Could you check a few things on this model? Use its own coordinates, in mm. A direction names the side the tool comes from. Coordinates: 2 decimals unless noted, no trailing zeros. Loops run counter-clockwise (first coordinate to the right, second up) from the corner with the lowest first, then second, coordinate; pieces in that order, holes last.
1) Imagine slicing it at D-D on x = -12. Please give me the cut outline in (y, z), plus the area to 3 significant figures.
2) For faces 1 (the face through (-19.962, 22.004, -21.009)), 2 (the face through (14.53, 63.57, -16.02)), 3 (the face through (39, 7, 17)), which set-ups out of +Z, -Z, +X, -X, +Y, -Y let a thin tool reach every point of the face, with its end or its side?
3) Will these pins go through, and if not, where does the flat tip stop? P1, Ø9.5, axis at x = -21, y = 24, coming from the +Z side; P2, Ø6.5, axis at x = 15, y = 60, coming from the +Z side; P3, Ø3.5, axis at x = 15, y = 60, coming from the +Z side.
4) Thinking about a two-plate mould opening in X: for faces 4 (the face through (39, 56, 17)), 5 (the face through (41, 39, 0)), 6 (the face through (-1, 49, 5)), which applies, released by +X, released by -X, zero draft, split by the parting line, or undercut?
5) Imagine slicing it at C-C on z = 4. Please give me the cut outline in (x, y), plus the area to 3 significant figures.
6) Imagine slicing it at B-B on x = 15. Please give me the cut outline in (y, z).
7) If I drill on line 1 along Y through (x, z) = (15, -20.8); line 2 along Y through (x, z) = (-31, 4); line 3 along X through (y, z) = (32.5, 10), over which ranges is the centre line in solid material (lowest first)?
8) Imagine slicing it at A-A on y = 60. Please give me the cut outline in (x, z), plus the area to 3 significant figures.
```python
from build123d import *

# Parameters (mm, degrees)
SKETCH_1_W          = 82
SKETCH_1_H          = 48
EXTRUDE_1_DEPTH     = 80
SKETCH_2_W          = 72
SKETCH_2_H          = 44
SKETCH_2_H_2        = 22
CUT_EXTRUDE_1_DEPTH = 38
CUT_EXTRUDE_2_REACH = 84
SKETCH_3_W          = 7
SKETCH_3_H          = 4
SKETCH_5_R          = 3.6
CUT_EXTRUDE_3_DEPTH = 4.1
CUT_EXTRUDE_4_REACH = 12
SKETCH_6_R          = 2.25


with BuildPart() as part:
    # 草圖1 → 填料-伸長1 (new body)
    with BuildSketch(Plane(origin=(0, 0, 0), x_dir=(1, 0, 0), z_dir=(0, 1, 0))):
        Rectangle(SKETCH_1_W, SKETCH_1_H)
    extrude(amount=EXTRUDE_1_DEPTH)

    # 草圖2 → 除料-伸長1 (cut)
    with BuildSketch(Plane.XY.offset(24)):
        with Locations((0, 27)):
            Rectangle(SKETCH_2_W, SKETCH_2_H)
        with Locations((0, 65)):
            Rectangle(SKETCH_2_W, SKETCH_2_H_2)
    extrude(amount=-CUT_EXTRUDE_1_DEPTH, mode=Mode.SUBTRACT)

    # 草圖3 → 除料-伸長2 (cut, up to next)
    with BuildSketch(Plane(origin=(41, 0, 0), x_dir=(0, 0, -1), z_dir=(1, 0, 0)), mode=Mode.PRIVATE) as cut_extrude_2_sk1:
        with Locations((-20.5, 7)):
            Rectangle(SKETCH_3_W, SKETCH_3_H)
    cut_extrude_2_tool1 = extrude(cut_extrude_2_sk1.sketch, amount=-CUT_EXTRUDE_2_REACH, mode=Mode.PRIVATE) & part.part
    add(cut_extrude_2_tool1.solids().sort_by_distance((41, 7, 20.5))[0], mode=Mode.SUBTRACT)
    # 草圖3 → 除料-伸長2 (cut, up to next)
    with BuildSketch(Plane(origin=(41, 0, 0), x_dir=(0, 0, -1), z_dir=(1, 0, 0)), mode=Mode.PRIVATE) as cut_extrude_2_sk2:
        with Locations((-20.5, 56)):
            Rectangle(SKETCH_3_W, SKETCH_3_H)
    cut_extrude_2_tool2 = extrude(cut_extrude_2_sk2.sketch, amount=-CUT_EXTRUDE_2_REACH, mode=Mode.PRIVATE) & part.part
    add(cut_extrude_2_tool2.solids().sort_by_distance((41, 56, 20.5))[0], mode=Mode.SUBTRACT)

    # 草圖5 → 除料-伸長3 (cut)
    with BuildSketch(Plane.XY.offset(-14)):
        with Locations((-21, 60)):
            Circle(SKETCH_5_R)
        with Locations((15, 60)):
            Circle(SKETCH_5_R)
        with Locations((15, 24)):
            Circle(SKETCH_5_R)
        with Locations((-21, 24)):
            Circle(SKETCH_5_R)
    extrude(amount=-CUT_EXTRUDE_3_DEPTH, mode=Mode.SUBTRACT)

    # 草圖6 → 除料-伸長4 (cut, up to next)
    with BuildSketch(Plane.XY.offset(-14), mode=Mode.PRIVATE) as cut_extrude_4_sk1:
        with Locations((-21, 60)):
            Circle(SKETCH_6_R)
    cut_extrude_4_tool1 = extrude(cut_extrude_4_sk1.sketch, amount=-CUT_EXTRUDE_4_REACH, mode=Mode.PRIVATE) & part.part
    add(cut_extrude_4_tool1.solids().sort_by_distance((-21, 60, -14))[0], mode=Mode.SUBTRACT)
    # 草圖6 → 除料-伸長4 (cut, up to next)
    with BuildSketch(Plane.XY.offset(-14), mode=Mode.PRIVATE) as cut_extrude_4_sk2:
        with Locations((15, 60)):
            Circle(SKETCH_6_R)
    cut_extrude_4_tool2 = extrude(cut_extrude_4_sk2.sketch, amount=-CUT_EXTRUDE_4_REACH, mode=Mode.PRIVATE) & part.part
    add(cut_extrude_4_tool2.solids().sort_by_distance((15, 60, -14))[0], mode=Mode.SUBTRACT)
    # 草圖6 → 除料-伸長4 (cut, up to next)
    with BuildSketch(Plane.XY.offset(-14), mode=Mode.PRIVATE) as cut_extrude_4_sk3:
        with Locations((15, 24)):
            Circle(SKETCH_6_R)
    cut_extrude_4_tool3 = extrude(cut_extrude_4_sk3.sketch, amount=-CUT_EXTRUDE_4_REACH, mode=Mode.PRIVATE) & part.part
    add(cut_extrude_4_tool3.solids().sort_by_distance((15, 24, -14))[0], mode=Mode.SUBTRACT)
    # 草圖6 → 除料-伸長4 (cut, up to next)
    with BuildSketch(Plane.XY.offset(-14), mode=Mode.PRIVATE) as cut_extrude_4_sk4:
        with Locations((-21, 24)):
            Circle(SKETCH_6_R)
    cut_extrude_4_tool4 = extrude(cut_extrude_4_sk4.sketch, amount=-CUT_EXTRUDE_4_REACH, mode=Mode.PRIVATE) & part.part
    add(cut_extrude_4_tool4.solids().sort_by_distance((-21, 24, -14))[0], mode=Mode.SUBTRACT)


solid = part.part
```
Filled in:
1. outline: (0, -24) - (80, -24) - (80, 24) - (76, 24) - (76, -14) - (54, -14) - (54, 24) - (49, 24) - (49, -14) - (5, -14) - (5, 24) - (0, 24) - close
1. area: 1,330 mm2
2. face 1: +Z, -Z
2. face 2: +Z
2. face 3: +Z, +X
3. P1: stops at z = -14
3. P2: stops at z = -18.1
3. P3: passes through
4. face 4: zero draft
4. face 5: released by +X
4. face 6: undercut
5. outline: (-41, 0) - (41, 0) - (41, 80) - (-41, 80) - close; hole (-36, 5) - (36, 5) - (36, 49) - (-36, 49) - close; hole (-36, 54) - (36, 54) - (36, 76) - (-36, 76) - close
5. area: 1,810 mm2
6. outline: (0, -24) - (21.75, -24) - (21.75, -18.1) - (20.4, -18.1) - (20.4, -14) - (5, -14) - (5, 24) - (0, 24) - close; (26.25, -24) - (57.75, -24) - (57.75, -18.1) - (56.4, -18.1) - (56.4, -14) - (54, -14) - (54, 24) - (49, 24) - (49, -14) - (27.6, -14) - (27.6, -18.1) - (26.25, -18.1) - close; (62.25, -24) - (80, -24) - (80, 24) - (76, 24) - (76, -14) - (63.6, -14) - (63.6, -18.1) - (62.25, -18.1) - close
7. line 1: y = 0 to 21.75, 26.25 to 57.75, 62.25 to 80
7. line 2: y = 0 to 5, 49 to 54, 76 to 80
7. line 3: x = -41 to -36, 36 to 41
8. outline: (-41, -24) - (-23.25, -24) - (-23.25, -18.1) - (-24.6, -18.1) - (-24.6, -14) - (-36, -14) - (-36, 24) - (-41, 24) - close; (-18.75, -24) - (12.75, -24) - (12.75, -18.1) - (11.4, -18.1) - (11.4, -14) - (-17.4, -14) - (-17.4, -18.1) - (-18.75, -18.1) - close; (17.25, -24) - (41, -24) - (41, 24) - (36, 24) - (36, -14) - (18.6, -14) - (18.6, -18.1) - (17.25, -18.1) - close
8. area: 1,090 mm2
